from build123d import *

# Parameters (mm, degrees)
BOSS_EXTRUDE1_DEPTH = 15
BOSS_EXTRUDE4_DEPTH = 15
SKETCH3_R           = 1
CUT_EXTRUDE1_DEPTH  = 25


with BuildPart() as part:
    # Sketch1 → Boss-Extrude1 (new body)
    with BuildSketch(Plane.XY):
        Polygon((0, 0), (38, 0), (38, 58), (33, 58), (33, 5), (0, 5), align=None)
    extrude(amount=BOSS_EXTRUDE1_DEPTH)

    # Sketch2 → Boss-Extrude4 (add)
    with BuildSketch(Plane.XY.offset(15)):
        with BuildLine():
            Line((33, 58), (26.937822174, 61.5))
            ThreePointArc((26.937822174, 61.5), (26.104169314, 65.983298832), (30.662536905, 66.110697479))
            Line((30.662536905, 66.110697479), (38, 58))
            Line((38, 58), (33, 58))
        make_face()
    extrude(amount=-BOSS_EXTRUDE4_DEPTH)

    # Sketch3 → Cut-Extrude1 (cut)
    with BuildSketch(Plane.XY.offset(15)):
        with Locations((28.437822174, 64.098076211)):
            Circle(SKETCH3_R)
    extrude(amount=-CUT_EXTRUDE1_DEPTH, mode=Mode.SUBTRACT)


solid = part.part
Geometry: final body of the model. Coordinates: model frame, mm. A direction names the side the tool comes from. Coordinates: 2 decimals unless noted, no trailing zeros. Write each loop counter-clockwise with the first axis right and the second up, starting at its lowest first coordinate (ties: lowest second). Pieces come first, ordered by that corner, then holes. Notation, with made-up numbers: (57, 14.5) - (87, 14.5) arc R33 ccw to (87, 48.5) - close; hole circle Ø7 at (71.5, 45). An arc over 180 degrees is marked (long way). Return JSON: item names as keys, results as strings.
Item 1: Section query C-C (x = 9.5). Output: boundary loops of the cut face in (y, z).
Completed:
{"outline": "(0, 0) - (5, 0) - (5, 15) - (0, 15) - close"}
Item 2: Line query: L1, parallel to Y at x = 28, z = 13.5; L2, parallel to Y at x = 24.5, z = 14.25; L3, parallel to X at y = 13.5, z = 13.5. Output: solid intervals per line, ascending.
Completed:
{"L1": "y = 0 to 5, 60.89 to 63.2, 65 to 67.07", "L2": "y = 0 to 5", "L3": "x = 33 to 38"}
Item 3: Reachability of faces 4 (the face through (30.011, 59.726, 7.605)), 5 (the face through (0, 3, 7)) from +Z, -Z, +X, -X, +Y, -Y: full face, straight path, thin tool, end or side. Return the list, or none.
Completed:
{"face 4": "+Z, -Z, -X", "face 5": "+Z, -Z, -X, +Y, -Y"}
Item 4: Pull-direction query (X, two-part tool) for faces 1 (the face through (38, 29, 7)), 2 (the face through (28.98, 64.94, 7.6)), 3 (the face through (33.2, 23.8, 0)); classes: +X half, -X half, draft (parallel to the pull), parting line (faces both ways), or undercut.
Completed:
{"face 1": "+X half", "face 2": "undercut", "face 3": "draft"}
Item 5: Section query B-B (x = 31.5). Output: boundary loops of the cut face in (y, z).
Completed:
{"outline": "(0, 0) - (5, 0) - (5, 15) - (0, 15) - close; (58.87, 0) - (65.18, 0) - (65.18, 15) - (58.87, 15) - close"}
Item 6: Section query A-A (z = 6). Output: boundary loops of the cut face in (x, y), and give its area (3 significant figures).
Completed:
{"outline": "(0, 0) - (38, 0) - (38, 58) - (30.66, 66.11) arc R3 ccw (long way) to (26.94, 61.5) - (33, 58) - (33, 5) - (0, 5) - close; hole circle Ø2 at (28.44, 64.1)", "area": "510 mm2"}
Item 7: Section query D-D (y = 19). Output: boundary loops of the cut face in (x, z), and give its area (3 significant figures).
Completed:
{"outline": "(33, 0) - (38, 0) - (38, 15) - (33, 15) - close", "area": "75.0 mm2"}
Item 8: Pin query (flat end, axial travel): pin 1 Ø1 at (y, z) = (34, 10.5) entering from -X; pin 2 Ø4 at (x, z) = (12, 2) entering from -Y. Return the tip coordinate at first contact, or that it passes through.
Completed:
{"pin 1": "stops at x = 33", "pin 2": "stops at y = 0"}
